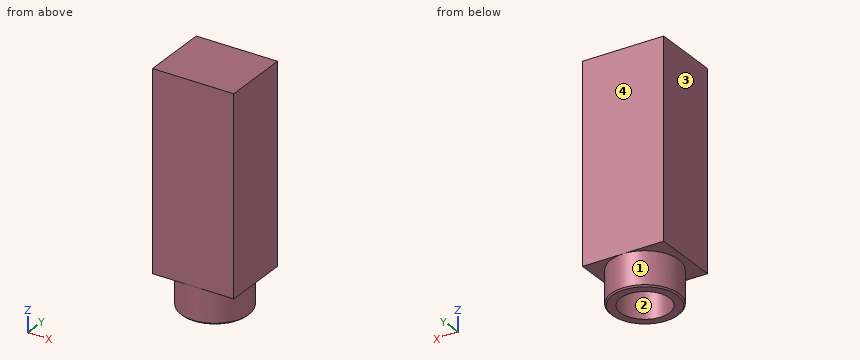
from build123d import *

# Parameters (mm, degrees)
SKETCH1_W           = 6
SKETCH1_H           = 5
BOSS_EXTRUDE1_DEPTH = 14.5
SKETCH2_R           = 2.5
BOSS_EXTRUDE2_DEPTH = 2.5
SKETCH3_R           = 1.8
CUT_EXTRUDE1_DEPTH  = 2.5
CHAMFER1_SIZE       = 0.1


with BuildPart() as part:
    # Sketch1 → Boss-Extrude1 (new body)
    with BuildSketch(Plane.XY):
        Rectangle(SKETCH1_W, SKETCH1_H)
    extrude(amount=BOSS_EXTRUDE1_DEPTH)

    # Sketch2 → Boss-Extrude2 (add)
    with BuildSketch(Plane(origin=(0, 0, 0), x_dir=(-1, 0, 0), z_dir=(0, 0, -1))):
        with Locations(Location((0, 0, 0), (0, 0, 270))):
            Circle(SKETCH2_R)
    extrude(amount=BOSS_EXTRUDE2_DEPTH)

    # Sketch3 → Cut-Extrude1 (cut)
    with BuildSketch(Plane(origin=(0, 0, -2.5), x_dir=(-1, 0, 0), z_dir=(0, 0, -1))):
        Circle(SKETCH3_R)
    extrude(amount=-CUT_EXTRUDE1_DEPTH, mode=Mode.SUBTRACT)

    # Chamfer1
    chamfer1_edges = [part.edges().sort_by_distance(p)[0] for p in [
        (0, 2.5, -2.5),
    ]]
    chamfer(chamfer1_edges, length=CHAMFER1_SIZE)


solid = part.part
Geometry: final body of the model. Coordinates: model frame, mm. Face numbers are marked on the shaded views. Give positions to 0.01 mm unless a question says otherwise; leave off trailing zeros. Order: outer loops, then holes, each group sorted by start corner. A loop starts at its lowest first (then second) coordinate and runs counter-clockwise, first axis right, second up. Notation, with made-up numbers: (70.5, 62) -> (86.5, 62) arc R35 ccw to (86.5, 101) -> close; hole circle Ø1 at (-7, -1.75). An arc over 180 degrees is marked (long way). Write each question's results on one line, items separated by ' | '.
1) Draft query along X for the marked faces 1, 2, 3 and 4. Return one class per face: released by +X, released by -X, zero draft, split by the parting line, or undercut.
Geometry says:
face 1: split by the parting line | face 2: undercut | face 3: released by -X | face 4: zero draft
2) Line query: line 1 along Z through (x, y) = (-0.2, -1.3); line 2 along Z through (x, y) = (2.05, 1.3). Output: solid intervals per line, ascending.
Geometry says:
line 1: z = 0 to 14.5 | line 2: z = -2.47 to 14.5
3) First-contact query: pin 1 Ø2 at (x, y) = (2, 1.5) entering from -Z. Flat tip, straight axial feed; report the tip coordinate or a pass-through.
Geometry says:
pin 1: stops at z = -2.5
4) Cut plane A-A (y = 0). Output: boundary loops of the cut face in (x, z), and give its area (3 significant figures).
Geometry says:
outline: (-3, 0) -> (-2.5, 0) -> (-2.5, -2.4) -> (-2.4, -2.5) -> (-1.8, -2.5) -> (-1.8, 0) -> (1.8, 0) -> (1.8, -2.5) -> (2.4, -2.5) -> (2.5, -2.4) -> (2.5, 0) -> (3, 0) -> (3, 14.5) -> (-3, 14.5) -> close | area: 90.5 mm²
